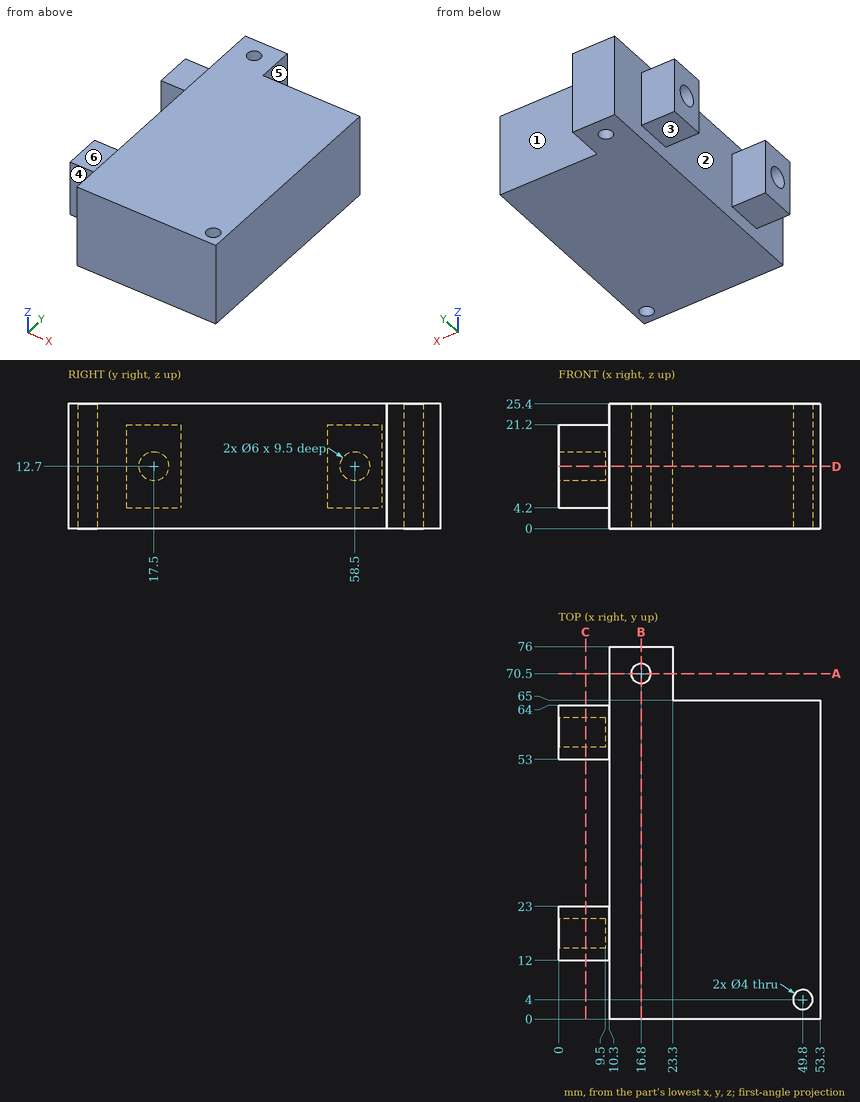
Answer from the drawing. Dimensions are ordinates in mm from the lowest x, y and z of the part. A direction names the side the tool comes from. Coordinates: 2 decimals unless noted, no trailing zeros. Order: outer loops, then holes, each group sorted by start corner. A loop starts at its lowest first (then second) coordinate and runs counter-clockwise, first axis right, second up. Notation, with made-up numbers: (27, -29) -> (70, -29) arc R33 ccw to (70, 0) -> close; hole circle Ø9 at (43, -37). An arc over 180 degrees is marked (long way). Answer as a JSON object with one key per item and string values.
1) Each of these flat-tipped pins is pushed along its axis until it touches: pin 1 (2 mm diameter, centred on y = 19, z = 22, fed in from -X); pin 2 (3 mm diameter, centred on x = 5.5, y = 18.5, fed in from +Z); pin 3 (4 mm diameter, centred on y = 36, z = 7, fed in from -X); pin 4 (5 mm diameter, centred on x = 7, z = 16, fed in from +Y). Where does it stop, or does it pass through?
Model answer:
{"pin 1": "stops at x = 0", "pin 2": "stops at z = 21.2", "pin 3": "stops at x = 10.3", "pin 4": "stops at y = 64"}
2) A tool of negligible diameter and unlimited length cuts with its end or side. For the marked faces 4, 5 and 6, from which of +Z, -Z, +X, -X, +Y, -Y can it reach the whole face along a straight path? Write none if from no direction.
Model answer:
{"face 4": "+Z, -Z, -X, -Y", "face 5": "+Z, -Z, +X, +Y", "face 6": "+Z, -X, +Y, -Y"}
3) A cutting plane is placed at A-A, the plane y = 70.5. Determine the outline of the cut face in (x, z), plus the area to 3 significant figures.
Model answer:
{"outline": "(10.3, 0) -> (14.8, 0) -> (14.8, 25.4) -> (10.3, 25.4) -> close; (18.8, 0) -> (23.3, 0) -> (23.3, 25.4) -> (18.8, 25.4) -> close", "area": "229 mm²"}
4) Consider line 1 along Y through (x, z) = (7.25, 12.7); line 2 along Y through (x, z) = (2, 10); line 3 along X through (y, z) = (56, 3.75). Determine where each line is inside the solid, lowest interval first. Write a range as from..to.
Model answer:
{"line 1": "y = 12..14.5, 20.5..23, 53..55.5, 61.5..64", "line 2": "y = 12..16.19, 18.81..23, 53..57.19, 59.81..64", "line 3": "x = 10.3..53.3"}
5) A cutting plane is placed at B-B, the plane x = 16.8. Determine the outline of the cut face in (y, z).
Model answer:
{"outline": "(0, 0) -> (68.5, 0) -> (68.5, 25.4) -> (0, 25.4) -> close; (72.5, 0) -> (76, 0) -> (76, 25.4) -> (72.5, 25.4) -> close"}
6) A cutting plane is placed at C-C, the plane x = 5.5. Determine the outline of the cut face in (y, z), plus the area to 3 significant figures.
Model answer:
{"outline": "(12, 4.2) -> (23, 4.2) -> (23, 21.2) -> (12, 21.2) -> close; (53, 4.2) -> (64, 4.2) -> (64, 21.2) -> (53, 21.2) -> close; hole circle Ø6 at (17.5, 12.7); hole circle Ø6 at (58.5, 12.7)", "area": "317 mm²"}
7) The mould has two halves that part along Y. Classify the marked faces 1, 2 and 3: released by +Y, released by -Y, zero draft, split by the parting line, or undercut.
Model answer:
{"face 1": "released by +Y", "face 2": "undercut", "face 3": "zero draft"}
8) A cutting plane is placed at D-D, the plane z = 12.7. Determine the outline of the cut face in (x, y).
Model answer:
{"outline": "(0, 12) -> (10.3, 12) -> (10.3, 0) -> (53.3, 0) -> (53.3, 65) -> (23.3, 65) -> (23.3, 76) -> (10.3, 76) -> (10.3, 64) -> (0, 64) -> (0, 61.5) -> (9.5, 61.5) -> (9.5, 55.5) -> (0, 55.5) -> (0, 53) -> (10.3, 53) -> (10.3, 23) -> (0, 23) -> (0, 20.5) -> (9.5, 20.5) -> (9.5, 14.5) -> (0, 14.5) -> close; hole circle Ø4 at (16.8, 70.5); hole circle Ø4 at (49.8, 4)"}
